Verification items for the finished model (mm, model axes). Face numbers are marked on the shaded views. A direction names the side the tool comes from. Round coordinates to 2 decimals unless told otherwise and drop trailing zeros. Write each loop counter-clockwise with the first axis right and the second up, starting at its lowest first coordinate (ties: lowest second). Pieces come first, ordered by that corner, then holes. Notation, with made-up numbers: M 74,55 L 131,55 A21 ccw 131,90 Z; hole C 45,-35 d8. An arc over 180 degrees is marked long. One line per item, written item: value. Start each with the question number.
Item 1: Section check B-B, the plane z = 15.1. Record the cut outline in (x, y), then the cut area to 3 significant figures.
Item 2: Thickness scan on probe 1 along Y at (x, z) = (95, 6.75); probe 2 along X at (y, z) = (37.5, 15.1); probe 3 along Z at (x, y) = (-25, 39). Record the ranges inside material, lowest first. Write a range as from..to.
Item 3: Tool access check on the marked faces 1, 2 and 3. Record the directions out of +Z, -Z, +X, -X, +Y, -Y that give a thin tool (end or side, any length) a straight path to the whole face; none if there is none.
Item 4: Section check A-A, the plane x = -25.4. Record the cut outline in (y, z).
Item 5: Section check D-D, the plane y = 17. Record the cut outline in (x, z), then the cut area to 3 significant figures.
Item 6: Section check C-C, the plane x = -4.5. Record the cut outline in (y, z).
Item 7: Gauge pin test, flat ends, axial feed: pin 1 (16 mm diameter, centred on x = 1, z = 18.5, fed in from +Y); pin 2 (5 mm diameter, centred on x = 12, z = 24.5, fed in from -Y); pin 3 (3.5 mm diameter, centred on x = -95, y = -46, fed in from -Z); pin 4 (11 mm diameter, centred on y = 41.5, z = 19.5, fed in from +X). Record the tip position at first contact, or that the pin passes through.
Autodesk Inventor part; units mm, degrees
ref_plane "YZ Plane" through (0, 0, 0) normal (1, 0, 0) x (0, 1, 0)
ref_plane "XZ Plane" through (0, 0, 0) normal (0, 1, 0) x (-1, 0, 0)
ref_plane "XY Plane" through (0, 0, 0) normal (0, 0, 1) x (1, 0, 0)
sketch "Sketch1" plane through (0, 0, 0) normal (0, 0, 1) x (1, 0, 0)
  line L0 (-100, 50) -> (100, 50)
  line L1 (100, 50) -> (100, -50)
  line L2 (100, -50) -> (-100, -50)
  line L3 (-100, -50) -> (-100, 50)
  point P0 (0, 0)
  point P1 (100, 0)
  point P2 (0, 50)
  dimension "d0" = 200
  dimension "d1" = 100
extrude "Extrusion1" add sketch "Sketch1" along normal blind 10
sketch "Sketch2" plane through (0, 0, 10) normal (0, 0, 1) x (1, 0, 0)
  line L0 (30.48, -9.53) -> (-30.48, -9.53)
  line L1 (-30.48, -9.53) -> (-30.48, 40)
  line L2 (-30.48, 40) -> (30.48, 40)
  line L3 (30.48, 40) -> (30.48, -9.53)
  circle A0 centre (25.4, 34.92) radius 2.15
  line L4 (100, 50) -> (-100, 50)
  circle A1 centre (25.4, -4.45) radius 2.15
  circle A2 centre (-25.4, -4.45) radius 2.15
  circle A3 centre (-25.4, 34.92) radius 2.15
  point P0 (0, 0)
  point P1 (0, -9.53)
  dimension "d4" = 60.96
  dimension "d5" = 49.53
  dimension "d6" = 4.3
  dimension "d7" = 5.08
  dimension "d8" = 5.08
  dimension "d9" = 10
  dimension "d10" = 5.08
  dimension "d11" = 5.08
  dimension "d12" = 4.3
  dimension "d13" = 4.3
  dimension "d14" = 5.08
  dimension "d15" = 5.08
  dimension "d16" = 5.08
  dimension "d17" = 5.08
  dimension "d18" = 4.3
extrude "Extrusion2" [suppressed]
sketch "Sketch3" plane through (0, 0, 10) normal (0, 0, 1) x (1, 0, 0)
  line L0 (98, -48) -> (28, -48)
  line L1 (28, -48) -> (28, -23)
  line L2 (28, -23) -> (98, -23)
  line L3 (98, -23) -> (98, -48)
  line L4 (-100, -50) -> (100, -50)
  line L5 (-100, 50) -> (-100, -50)
  line L6 (100, -50) -> (100, 50)
  circle A0 centre (95, -46) radius 1.4
  circle A1 centre (95, -35.5) radius 1.4
  circle A2 centre (34, -46) radius 1.4
  circle A3 centre (34, -35.5) radius 1.4
  line L7 (0, 0) -> (0, -50) construction
  circle A4 centre (-95, -46) radius 1.4
  circle A5 centre (-95, -35.5) radius 1.4
  circle A6 centre (-34, -46) radius 1.4
  circle A7 centre (-34, -35.5) radius 1.4
  dimension "d21" = 70
  dimension "d22" = 25
  dimension "d25" = 2
  dimension "d27" = 2
  dimension "d28" = 2.8
  dimension "d31" = 2.8
  dimension "d38" = 2.8
  dimension "d39" = 2.8
  dimension "d42" = 10.5
  dimension "d43" = 10.5
  dimension "d44" = 61
  dimension "d45" = 3
  dimension "d49" = 4
extrude "Extrusion4" cut sketch "Sketch3" against normal up to surface (10 mm away) contours A0 | A1 | A2 | A3 | A4 | A5 | A6 | A7
sketch "Sketch4" plane through (0, 0, 10) normal (0, 0, 1) x (1, 0, 0)
  line L0 (35, 35) -> (-35, 35)
  line L1 (-35, 35) -> (-35, 45)
  line L2 (-35, 45) -> (35, 45)
  line L3 (35, 45) -> (35, 35)
  line L4 (-100, -50) -> (100, -50)
  point P0 (0, 0)
  point P1 (0, 35)
  dimension "d50" = 85
  dimension "d51" = 10
  dimension "d52" = 70
extrude "Extrusion5" add sketch "Sketch4" along normal blind 20
sketch "Sketch5" plane through (-100, 50, 0) normal (0, 1, 0) x (1, 0, 0)
  line L0 (130.48, -30.7809) -> (69.52, -30.7809)
  line L1 (69.52, -30.7809) -> (69.52, -15.7809)
  line L2 (69.52, -15.7809) -> (130.48, -15.7809)
  line L3 (130.48, -15.7809) -> (130.48, -30.7809)
  line L4 (0, 0) -> (200, 0)
  circle A0 centre (125.4, -15.1) radius 2.15
  circle A1 centre (74.6, -15.1) radius 2.15
  line L5 (200, -10) -> (135, -10)
  line L6 (65, -10) -> (0, -10)
  point P0 (100, 0)
  point P1 (100, 0)
  point P2 (100, -30.7809)
  dimension "d55" = 60.96
  dimension "d56" = 15
  dimension "d57" = 4.3
  dimension "d58" = 4.3
  dimension "d59" = 5.1
  dimension "d60" = 5.1
  dimension "d61" = 5.08
  dimension "d62" = 5.08
extrude "Extrusion6" cut sketch "Sketch5" against normal up to surface (15 mm away) contours A0 L2 | L2 A0 | A1 L2 | L2 A1
properties part number "motor holder"
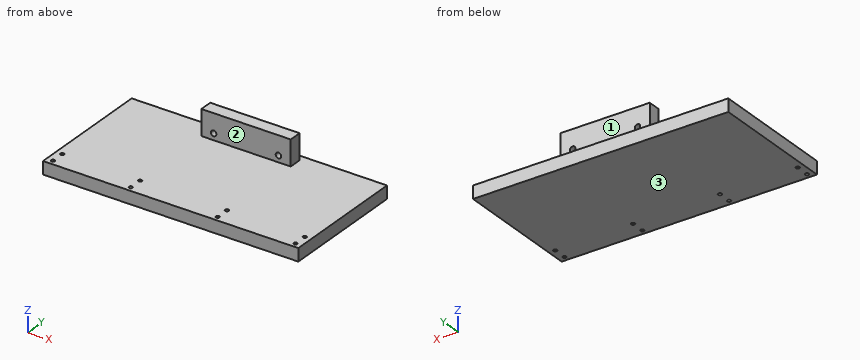
Response values:
1. outline: M -35,35 L -27.55,35 L -27.55,45 L -35,45 Z; M -23.25,35 L 23.25,35 L 23.25,45 L -23.25,45 Z; M 27.55,35 L 35,35 L 35,45 L 27.55,45 Z
1. area: 614 mm2
2. probe 1: y = -50..-47.4, -44.6..-36.9, -34.1..50
2. probe 2: x = -35..-27.55, -23.25..23.25, 27.55..35
2. probe 3: z = 0..12.99, 17.21..30
3. face 1: +Z, +X, -X, +Y
3. face 2: +Z, +X, -X, -Y
3. face 3: -Z, +X, -X, +Y, -Y
4. outline: M -50,0 L 50,0 L 50,10 L 45,10 L 45,12.95 L 35,12.95 L 35,10 L -50,10 Z; M 35,17.25 L 45,17.25 L 45,30 L 35,30 Z
5. outline: M -100,0 L 100,0 L 100,10 L -100,10 Z
5. area: 2,000 mm2
6. outline: M -50,0 L 50,0 L 50,10 L 45,10 L 45,30 L 35,30 L 35,10 L -50,10 Z
7. pin 1: stops at y = 45
7. pin 2: stops at y = 35
7. pin 3: stops at z = 0
7. pin 4: stops at x = 35
